Design review of the part built by this model. Coordinates are the model's own, in mm. Face numbers are marked on the shaded views. A direction names the side the tool comes from. Coordinates: 2 decimals unless noted, no trailing zeros. Order: outer loops, then holes, each group sorted by start corner. A loop starts at its lowest first (then second) coordinate and runs counter-clockwise, first axis right, second up. Notation, with made-up numbers: M 21,-39.5 L 51,-39.5 A26 ccw 51,-17.5 Z; hole C -32,32 d10. An arc over 180 degrees is marked long. Answer in a Markdown table with one row per item.
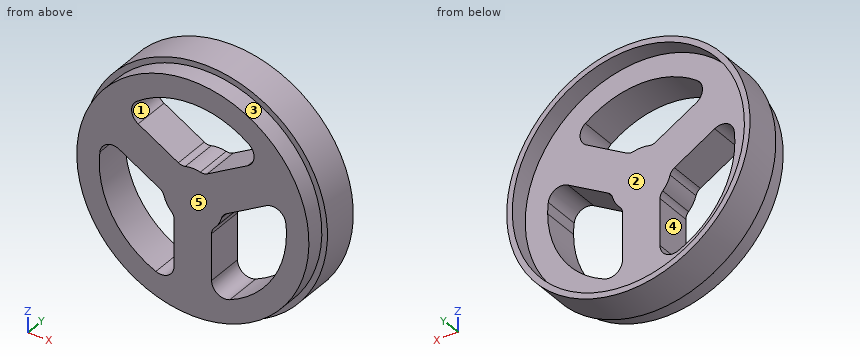
from build123d import *

# Parameters (mm, degrees)
CUT_EXTRUDE1_DEPTH = 20
FILLET1_R          = 5
FILLET2_R          = 7


with BuildPart() as part:
    # Sketch1 → Revolve1 (revolve)
    with BuildSketch(Plane.XY, mode=Mode.PRIVATE) as revolve1_sk:
        Polygon((0, 0), (-62, 0), (-62, 10), (-65, 10), (-65, 30), (-62, 30), (-62, 20), (0, 20), align=None)
    revolve(revolve1_sk.sketch.rotate(Axis((0, 0, 0), (0, 1, 0)), 270), axis=Axis((0, 0, 0), (0, 1, 0)))

    # Szkic1 → Cut-Extrude1 (cut)
    with BuildSketch(Plane(origin=(0, 0, 0), x_dir=(1, 0, 0), z_dir=(0, 1, 0))):
        with BuildLine():
            ThreePointArc((-15.816653826, 2.415256039), (-13.856406461, 8), (-10, 12.489995997))
            Line((-10, 12.489995997), (-10, 48.989794856))
            ThreePointArc((-10, 48.989794856), (-43.301270189, 25), (-47.426406871, -15.83464339))
            Line((-47.426406871, -15.83464339), (-15.816653826, 2.415256039))
        make_face()
        with BuildLine():
            Line((10, 48.989794856), (10, 12.489995997))
            ThreePointArc((10, 12.489995997), (13.856406461, 8), (15.816653826, 2.415256039))
            Line((15.816653826, 2.415256039), (47.426406871, -15.83464339))
            ThreePointArc((47.426406871, -15.83464339), (49.352407963, -8.021211144), (50, 0))
            ThreePointArc((50, 0), (38.729833462, 31.622776602), (10, 48.989794856))
        make_face()
        with BuildLine():
            ThreePointArc((5.816653826, -14.905252036), (0, -16), (-5.816653826, -14.905252036))
            Line((-5.816653826, -14.905252036), (-37.426406871, -33.155151466))
            ThreePointArc((-37.426406871, -33.155151466), (0, -50), (37.426406871, -33.155151466))
            Line((37.426406871, -33.155151466), (5.816653826, -14.905252036))
        make_face()
    extrude(amount=CUT_EXTRUDE1_DEPTH, mode=Mode.SUBTRACT)

    # Fillet1
    fillet1_edges = [part.edges().sort_by_distance(p)[0] for p in [
        (10, 10, -12.489995997),
        (15.816653826, 10, -2.415256039),
        (5.816653826, 10, 14.905252036),
        (-5.816653826, 10, 14.905252036),
        (-15.816653826, 10, -2.415256039),
        (-10, 10, -12.489995997),
    ]]
    fillet(fillet1_edges, radius=FILLET1_R)

    # Fillet2
    fillet2_edges = [part.edges().sort_by_distance(p)[0] for p in [
        (47.426406871, 10, 15.83464339),
        (10, 10, -48.989794856),
        (-37.426406871, 10, 33.155151466),
        (37.426406871, 10, 33.155151466),
        (-10, 10, -48.989794856),
        (-47.426406871, 10, 15.83464339),
    ]]
    fillet(fillet2_edges, radius=FILLET2_R)


solid = part.part
(1) Add section C-C, the plane y = 14.25. Give the boundary of the cut face in (x, z), and give its area (3 significant figures).
Return value:
| item | result |
|---|---|
| outline | C 0,0 d130; hole M -49.66,5.84 A50 ccw -19.77,-45.93 A7 ccw -10,-39.5 L -10,-14.7 A5 ccw -11.43,-11.2 A16 cw -15.41,-4.3 A5 ccw -17.73,-1.31 L -39.21,11.09 A7 ccw Z; hole M -29.89,40.08 A7 ccw -29.21,28.41 L -7.73,16.01 A5 ccw -3.98,15.5 A16 cw 3.98,15.5 A5 ccw 7.73,16.01 L 29.21,28.41 A7 ccw 29.89,40.08 A50 ccw Z; hole M 10,-39.5 A7 ccw 19.77,-45.93 A50 ccw 49.66,5.84 A7 ccw 39.21,11.09 L 17.73,-1.31 A5 ccw 15.41,-4.3 A16 cw 11.43,-11.2 A5 ccw 10,-14.7 Z |
| area | 8,450 mm2 |
(2) Insertion check: pin 1 Ø2 at (y, z) = (20.5, 51.5) entering from +X; pin 2 Ø12 at (x, y) = (-14, 16.5) entering from +Z; pin 3 Ø10 at (y, z) = (10.5, -29) entering from -X. Each pin has a flat end and moves straight along its axis. Give the tip position at first contact, or say it passes through.
Return value:
| item | result |
|---|---|
| pin 1 | stops at x = 40.92 |
| pin 2 | stops at z = 64.51 |
| pin 3 | stops at x = -60.41 |
(3) Add section A-A, the plane x = 0. Give the boundary of the cut face in (y, z).
Return value:
| item | result |
|---|---|
| outline | M 0,-62 L 10,-62 L 10,-65 L 30,-65 L 30,-62 L 20,-62 L 20,16 L 0,16 Z; M 0,50 L 20,50 L 20,62 L 30,62 L 30,65 L 10,65 L 10,62 L 0,62 Z |
(4) Draft analysis for pull direction X (two halves, no side actions). For the marked faces 3, 4 and 5, state which applies: pulls with the +X half, pulls with the -X half, needs draft (parallel to the pull), parting line crosses it, or undercut.
Return value:
| item | result |
|---|---|
| face 3 | parting line crosses it |
| face 4 | undercut |
| face 5 | needs draft |
(5) For the marked faces 1 and 2, list the 3-axis set-ups (+Z, -Z, +X, -X, +Y, -Y) from which the entire face can be reached by the end or side of a thin tool; tool diameter is ignored.
Return value:
| item | result |
|---|---|
| face 1 | +Y, -Y |
| face 2 | +Y |
(6) For line 1 along X through (y, z) = (25, 0); line 2 along X through (y, z) = (17.5, -2.5); line 3 along Z through (x, y) = (-12, 18.75), list the stretches that pass through material, from the lowest coordinate up. Write a range as from..to.
Return value:
| item | result |
|---|---|
| line 1 | x = -65..-62, 62..65 |
| line 2 | x = -64.95..-49.94, -16.34..16.34, 49.94..64.95 |
| line 3 | z = -63.88..-44.4, -10.58..18.48, 48.54..63.88 |
(7) Add section B-B, the plane z = 24.5. Give the boundary of the cut face in (x, y), and give its area (3 significant figures).
Return value:
| item | result |
|---|---|
| outline | M -60.21,10 L -56.95,10 L -56.95,0 L -22.44,0 L -22.44,20 L -56.95,20 L -56.95,30 L -60.21,30 Z; M 22.44,0 L 56.95,0 L 56.95,10 L 60.21,10 L 60.21,30 L 56.95,30 L 56.95,20 L 22.44,20 Z |
| area | 1,510 mm2 |
(8) Add section D-D, the plane z = 3. Give the boundary of the cut face in (x, y).
Return value:
| item | result |
|---|---|
| outline | M -64.93,10 L -61.93,10 L -61.93,0 L -49.91,0 L -49.91,20 L -61.93,20 L -61.93,30 L -64.93,30 Z; M -25.2,0 L 25.2,0 L 25.2,20 L -25.2,20 Z; M 49.91,0 L 61.93,0 L 61.93,10 L 64.93,10 L 64.93,30 L 61.93,30 L 61.93,20 L 49.91,20 Z |
